from build123d import *

# Parameters (mm, degrees)
SKETCH_1_R          = 50
SKETCH_1_R_2        = 7.5
EXTRUDE_2_DEPTH     = 20
SKETCH_4_R          = 40
CUT_EXTRUDE_1_DEPTH = 4
SKETCH_6_R          = 30
EXTRUDE_5_DEPTH     = 15
SKETCH_8_R          = 25
SKETCH_8_R_2        = 15
EXTRUDE_6_DEPTH     = 11
EXTRUDE_7_DEPTH     = 11
CUT_EXTRUDE_START   = 11
CUT_EXTRUDE_2_DEPTH = 6
CUT_EXTRUDE_START_2 = -6
CUT_EXTRUDE_3_DEPTH = 6


with BuildPart() as part:
    # Sketch 1 → Extrude 2 (new, symmetric)
    with BuildSketch(Plane(origin=(0, 0, 0), x_dir=(1, 0, 0), z_dir=(0, 1, 0))):
        with Locations(Location((0, 0, 0), (0, 0, 270))):
            Circle(SKETCH_1_R)
        with Locations(Location((-25, 0, 0), (0, 0, 270))):
            Circle(SKETCH_1_R_2, mode=Mode.SUBTRACT)
        with Locations(Location((-15.587245046, 19.545787062, 0), (0, 0, 270))):
            Circle(SKETCH_1_R_2, mode=Mode.SUBTRACT)
        with Locations(Location((5.563023349, 24.373197805, 0), (0, 0, 270))):
            Circle(SKETCH_1_R_2, mode=Mode.SUBTRACT)
        with Locations(Location((22.524221698, 10.847093478, 0), (0, 0, 270))):
            Circle(SKETCH_1_R_2, mode=Mode.SUBTRACT)
        with Locations(Location((22.524221698, -10.847093478, 0), (0, 0, 270))):
            Circle(SKETCH_1_R_2, mode=Mode.SUBTRACT)
        with Locations(Location((5.563023349, -24.373197805, 0), (0, 0, 270))):
            Circle(SKETCH_1_R_2, mode=Mode.SUBTRACT)
        with Locations(Location((-15.587245046, -19.545787062, 0), (0, 0, 270))):
            Circle(SKETCH_1_R_2, mode=Mode.SUBTRACT)
    extrude(amount=EXTRUDE_2_DEPTH, both=True)

    # Sketch 4 → Cut-Extrude 1 (cut)
    with BuildSketch(Plane(origin=(0, 20, 0), x_dir=(1, 0, 0), z_dir=(0, 1, 0))):
        with Locations(Location((0, 0, 0), (0, 0, 270))):
            Circle(SKETCH_4_R)
    cut_extrude_1 = extrude(amount=-CUT_EXTRUDE_1_DEPTH, mode=Mode.SUBTRACT)

    # Mirror 1: Cut-Extrude 1 across plane
    add(cut_extrude_1.mirror(Plane.ZX), mode=Mode.SUBTRACT)



with BuildPart() as body_2:
    # Sketch 6 → Extrude 5 (new, symmetric)
    with BuildSketch(Plane(origin=(0, 0, 0), x_dir=(1, 0, 0), z_dir=(0, 1, 0))):
        with Locations(Location((-110, 0, 0), (0, 0, 270))):
            Circle(SKETCH_6_R)
        Polygon((-92.679491924, 0), (-101.339745962, 15), (-118.660254038, 15), (-127.320508076, 0), (-118.660254038, -15), (-101.339745962, -15), align=None, mode=Mode.SUBTRACT)
    extrude(amount=EXTRUDE_5_DEPTH, both=True)


with BuildPart() as body_3:
    # Sketch 8 → Extrude 6 (new, symmetric)
    with BuildSketch(Plane(origin=(0, 0, 0), x_dir=(1, 0, 0), z_dir=(0, 1, 0))):
        with Locations(Location((106.066017178, -106.066017178, 0), (0, 0, 270))):
            Circle(SKETCH_8_R)
        with Locations(Location((106.066017178, -106.066017178, 0), (0, 0, 270))):
            Circle(SKETCH_8_R_2, mode=Mode.SUBTRACT)
    extrude(amount=EXTRUDE_6_DEPTH, both=True)


with BuildPart() as part_1:
    add(part.part)

    add(body_2.part)  # Extrude 7 merges body 2

    add(body_3.part)  # Extrude 7 merges body 3
    # Sketch 9 → Extrude 7 (add, symmetric)
    with BuildSketch(Plane(origin=(0, 0, 0), x_dir=(1, 0, 0), z_dir=(0, 1, 0))):
        with BuildLine():
            Line((-9.330441424, 49.121714779), (-110, 30))
            ThreePointArc((-110, 30), (-88.786796564, 21.213203436), (-80, 0))
            ThreePointArc((-80, 0), (-88.71993646, -21.146131933), (-109.810593048, -29.999402077))
            ThreePointArc((-109.810593048, -29.999402077), (-63.064827616, -34.060904943), (-17.875950367, -46.695293108))
            ThreePointArc((-17.875950367, -46.695293108), (-49.802326137, 4.44165637), (-9.330441424, 49.121714779))
        make_face()
        with BuildLine():
            Line((126.442712652, -91.581878213), (40.753390949, 28.968277929))
            ThreePointArc((40.753390949, 28.968277929), (47.632287093, 15.204118727), (50, 0))
            ThreePointArc((50, 0), (28.33904093, -41.19343102), (-17.875950367, -46.695293108))
            ThreePointArc((-17.875950367, -46.695293108), (39.329861169, -77.545156319), (86.774183491, -121.966493681))
            ThreePointArc((86.774183491, -121.966493681), (90.864028968, -86.219114285), (126.442712652, -91.581878213))
        make_face()
    extrude(amount=EXTRUDE_7_DEPTH, both=True)

    # Sketch 10 → Cut-Extrude 2 (cut)
    with BuildSketch(Plane(origin=(0, 0, 0), x_dir=(1, 0, 0), z_dir=(0, 1, 0)).offset(CUT_EXTRUDE_START)):
        with BuildLine():
            ThreePointArc((-43.829514678, 24.061871148), (-49.930321788, 2.638743289), (-46.121552708, -19.308090941))
            ThreePointArc((-46.121552708, -19.308090941), (-46.894642878, -24.442270002), (-51.807391271, -26.122259963))
            ThreePointArc((-51.807391271, -26.122259963), (-65.699920333, -23.457746699), (-79.715740029, -21.544949554))
            ThreePointArc((-79.715740029, -21.544949554), (-83.598085675, -18.902773341), (-83.577090418, -14.206683259))
            ThreePointArc((-83.577090418, -14.206683259), (-80.054612182, 1.80935028), (-85.479855197, 17.284747578))
            ThreePointArc((-85.479855197, 17.284747578), (-86.028032441, 22.041171589), (-82.326208539, 25.077710319))
            Line((-82.326208539, 25.077710319), (-49.145510288, 31.38022974))
            ThreePointArc((-49.145510288, 31.38022974), (-44.167091223, 29.4065854), (-43.829514678, 24.061871148))
        make_face()
        with BuildLine():
            ThreePointArc((99.202471828, -82.026638126), (90.358856707, -86.616464228), (84.010192893, -94.295689438))
            ThreePointArc((84.010192893, -94.295689438), (80.353400569, -96.884388509), (76.090892576, -95.504345545))
            ThreePointArc((76.090892576, -95.504345545), (49.969670312, -72.96331305), (21.11948881, -54.040220653))
            ThreePointArc((21.11948881, -54.040220653), (18.584494671, -49.509076454), (21.437529998, -45.171144635))
            ThreePointArc((21.437529998, -45.171144635), (38.390543683, -32.033828303), (48.279793254, -13.002367605))
            ThreePointArc((48.279793254, -13.002367605), (52.22522368, -9.381109934), (57.183111675, -11.405776572))
            Line((57.183111675, -11.405776572), (101.905101852, -74.321934522))
            ThreePointArc((101.905101852, -74.321934522), (102.547910869, -78.873778446), (99.202471828, -82.026638126))
        make_face()
    extrude(amount=-CUT_EXTRUDE_2_DEPTH, mode=Mode.SUBTRACT)

    # Sketch 11 → Cut-Extrude 3 (cut)
    with BuildSketch(Plane.XZ.offset(11).offset(CUT_EXTRUDE_START_2)):
        with BuildLine():
            Line((101.905101852, 74.321934522), (57.183111675, 11.405776572))
            ThreePointArc((57.183111675, 11.405776572), (52.22522368, 9.381109934), (48.279793254, 13.002367605))
            ThreePointArc((48.279793254, 13.002367605), (38.390543683, 32.033828303), (21.437529998, 45.171144635))
            ThreePointArc((21.437529998, 45.171144635), (18.584494671, 49.509076454), (21.11948881, 54.040220653))
            ThreePointArc((21.11948881, 54.040220653), (49.969670312, 72.96331305), (76.090892576, 95.504345545))
            ThreePointArc((76.090892576, 95.504345545), (80.353400569, 96.884388509), (84.010192893, 94.295689438))
            ThreePointArc((84.010192893, 94.295689438), (90.358856707, 86.616464228), (99.202471828, 82.026638126))
            ThreePointArc((99.202471828, 82.026638126), (102.547910869, 78.873778446), (101.905101852, 74.321934522))
        make_face()
        with BuildLine():
            Line((-49.145510288, -31.38022974), (-82.326208539, -25.077710319))
            ThreePointArc((-82.326208539, -25.077710319), (-86.028032441, -22.041171589), (-85.479855197, -17.284747578))
            ThreePointArc((-85.479855197, -17.284747578), (-80.054612182, -1.80935028), (-83.577090418, 14.206683259))
            ThreePointArc((-83.577090418, 14.206683259), (-83.598085675, 18.902773341), (-79.715740029, 21.544949554))
            ThreePointArc((-79.715740029, 21.544949554), (-65.699920333, 23.457746699), (-51.807391271, 26.122259963))
            ThreePointArc((-51.807391271, 26.122259963), (-46.894642878, 24.442270002), (-46.121552708, 19.308090941))
            ThreePointArc((-46.121552708, 19.308090941), (-49.930321788, -2.638743289), (-43.829514678, -24.061871148))
            ThreePointArc((-43.829514678, -24.061871148), (-44.167091223, -29.4065854), (-49.145510288, -31.38022974))
        make_face()
    extrude(amount=CUT_EXTRUDE_3_DEPTH, mode=Mode.SUBTRACT)


solid = part_1.part
Read the model definition and answer for the solid it produces. Units are mm, in the model's axes. A direction names the side the tool comes from. Give positions to 0.01 mm unless a question says otherwise; leave off trailing zeros. Write each loop counter-clockwise with the first axis right and the second up, starting at its lowest first coordinate (ties: lowest second). Pieces come first, ordered by that corner, then holes. Notation, with made-up numbers: (-32, 72.25) - (19, 72.25) arc R21 ccw to (19, 109.25) - close; hole circle Ø11 at (-0.75, 83). An arc over 180 degrees is marked (long way). Answer in a Markdown table with one row per item. Add a question column.
Item 1: A tool of negligible diameter and unlimited length cuts with its end or side. For faces 3 (the face through (61, -5, 54)), 4 (the face through (-64, 11, -34)), 5 (the face through (-110, 0, -15)), 6 (the face through (61, 5, 53)), from which of +Z, -Z, +X, -X, +Y, -Y can it reach the whole face along a straight path? Write none if from no direction.
Item 2: Find the intervals of material crossed by L1, parallel to Z at x = -108.5, y = -14; L2, parallel to X at y = -3, z = -5; L3, parallel to Z at x = 97.5, y = 9, in increasing order.
Item 3: Section D-D, the plane x = -61.5 is taken. Write down the section's boundary in (y, z).
Item 4: Flat-ended cylindrical pins translate along their axes: P1, Ø2, axis at y = -5, z = 106, coming from the -X side; P2, Ø10, axis at x = -83, y = 11, coming from the -Z side; P3, Ø1, axis at y = -4, z = 58, coming from the -X side. Find the tip coordinate at first contact, or state that the pin passes through.
Item 5: Section B-B, the plane x = 96 is taken. Write down the section's boundary in (y, z), and give its area (3 significant figures).
Item 6: Determine the mould class of faces 1 (the face through (-97.07, 0.21, 7.605)), 2 (the face through (-96, -15, -7)) for opening direction X: pulls with the +X half, pulls with the -X half, needs draft (parallel to the pull), parting line crosses it, or undercut.
Item 7: Section A-A, the plane z = 112.5 is taken. Write down the section's boundary in (x, y), and give its area (3 significant figures).
Item 8: Section C-C, the plane y = 2 is taken. Count the separate pieces of the cut face and the enclosed holes in it, and give its area (3 significant figures).
Recorded:
| question | item | result |
|---|---|---|
| 1 | face 3 | -Y |
| 1 | face 4 | -Z, +Y |
| 1 | face 5 | +Y, -Y |
| 1 | face 6 | +Y |
| 2 | L1 | z = -29.96 to -15, 15 to 29.96 |
| 2 | L2 | x = -139.58 to -124.43, -95.57 to -30.59, -19.41 to 17.83, 27.22 to 57.79 |
| 2 | L3 | z = 50.86 to 68.12, 82.58 to 93.75, 118.38 to 129.55 |
| 3 | outline | (-11, -39.21) - (11, -39.21) - (11, -29.03) - (5, -29.03) - (5, 24.18) - (11, 24.18) - (11, 34.35) - (-11, 34.35) - (-11, 24.18) - (-5, 24.18) - (-5, -29.03) - (-11, -29.03) - close |
| 4 | P1 | stops at x = 71.45 |
| 4 | P2 | stops at z = -36.08 |
| 4 | P3 | stops at x = 6.43 |
| 5 | outline | (-11, 48.75) - (11, 48.75) - (11, 66.01) - (5, 66.01) - (5, 83.18) - (11, 83.18) - (11, 94.95) - (-11, 94.95) - (-11, 83.18) - (-5, 83.18) - (-5, 66.01) - (-11, 66.01) - close; (-11, 117.19) - (11, 117.19) - (11, 128.95) - (-11, 128.95) - close |
| 5 | area | 1,070 mm2 |
| 6 | face 1 | undercut |
| 6 | face 2 | needs draft |
| 7 | outline | (78.57, -11) - (92.52, -11) - (92.52, 11) - (78.57, 11) - close; (119.62, -11) - (130.22, -11) - (130.22, 11) - (119.62, 11) - close |
| 7 | area | 540 mm2 |
| 8 | separate pieces | 1 |
| 8 | enclosed holes | 9 |
| 8 | area | 18,800 mm2 |
